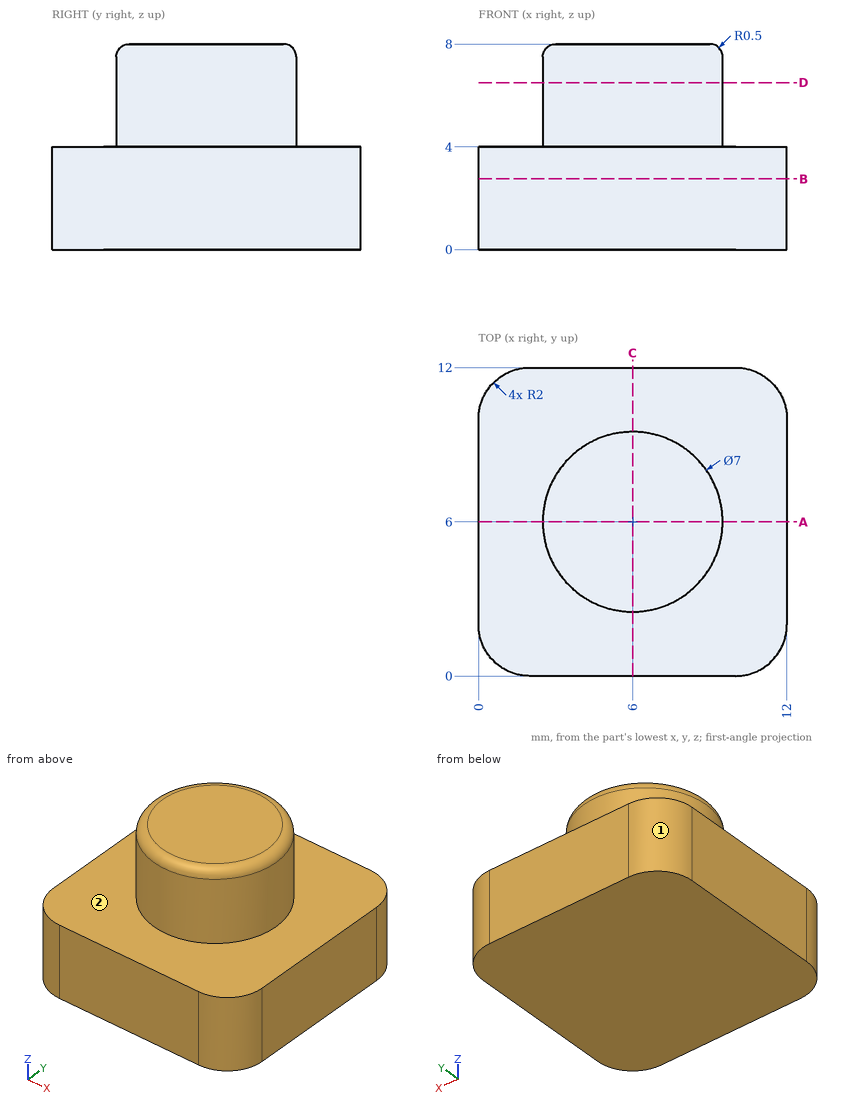
Source: three-view drawing plus pictorial views. Frame: mm from the lowest corner of the part. A direction names the side the tool comes from. Round coordinates to 2 decimals unless told otherwise and drop trailing zeros. Loops run counter-clockwise (first coordinate to the right, second up) from the corner with the lowest first, then second, coordinate; pieces in that order, holes last. Notation, with made-up numbers: M -23,2 L 17,2 A24 cw 17,23 Z; hole C 67.25,-35.75 d1. An arc over 180 degrees is marked long. Put each result on its own line as item: value.
(1) Section B-B, the plane z = 2.75. Return loops of the section in (x, y).
Solutions:
outline: M 0,2 A2 ccw 2,0 L 10,0 A2 ccw 12,2 L 12,10 A2 ccw 10,12 L 2,12 A2 ccw 0,10 Z
(2) Section D-D, the plane z = 6.5. Return loops of the section in (x, y), and give its area (3 significant figures).
Solutions:
outline: C 6,6 d7
area: 38.5 mm²
(3) Ray query, line 1 (Z direction, x = 9.5, y = 1.75); line 2 (Y direction, x = 10.5, z = 3.5); line 3 (X direction, y = 5.5, z = 4.5). Return the intervals inside material, ascending. Write a range as [from, to].
Solutions:
line 1: [0, 4]
line 2: [0.06, 11.94]
line 3: [2.54, 9.46]
(4) First-contact query: pin 1 (3 mm diameter, centred on x = 6.5, z = 6, fed in from -Y); pin 2 (1.5 mm diameter, centred on x = 10, y = 5.5, fed in from +Z). Flat tips, straight axial feed; report the tip coordinate or a pass-through.
Solutions:
pin 1: y = 2.5
pin 2: z = 7.91
(5) Access query for the marked faces 1 and 2. Directions: +Z, -Z, +X, -X, +Y, -Y. A direction counts if a zero-diameter tool reaches every point of the face in a straight line with its end or side. Return the directions, or none.
Solutions:
face 1: +Z, -Z, -X, +Y
face 2: +Z
(6) Section A-A, the plane y = 6. Return loops of the section in (x, z), and give its area (3 significant figures).
Solutions:
outline: M 0,0 L 12,0 L 12,4 L 9.5,4 L 9.5,7.5 A0.5 ccw 9,8 L 3,8 A0.5 ccw 2.5,7.5 L 2.5,4 L 0,4 Z
area: 75.9 mm²
